```python
from build123d import *

# Parameters (mm, degrees)
BOSS_EXTRUDE1_DEPTH = 10
SKETCH4_R           = 1.75
CUT_EXTRUDE3_DEPTH  = 10
SKETCH6_R           = 2
CUT_EXTRUDE5_DEPTH  = 2
CUT_EXTRUDE6_DEPTH  = 29.447319733
SKETCH8_W           = 5
SKETCH8_H           = 4.5
SKETCH8_W_2         = 1
SKETCH8_H_2         = 7
CUT_EXTRUDE7_DEPTH  = 5
CUT_EXTRUDE8_DEPTH  = 9
FILLET6_R           = 0.5


with BuildPart() as part:
    # Sketch1 → Boss-Extrude1 (new body)
    with BuildSketch(Plane(origin=(0, 0, 0), x_dir=(1, 0, 0), z_dir=(0, 1, 0))):
        Polygon((0, 0), (17, 0), (17, -20.5), (12, -20.5), (12, -16), (1, -16), (1, -7), (0, -7), align=None)
    extrude(amount=BOSS_EXTRUDE1_DEPTH)

    # Sketch4 → Cut-Extrude3 (cut)
    with BuildSketch(Plane(origin=(0, 10, 0), x_dir=(1, 0, 0), z_dir=(0, 1, 0))):
        with Locations(Location((6, -11, 0), (0, 0, 270))):
            Circle(SKETCH4_R)
    extrude(amount=-CUT_EXTRUDE3_DEPTH, mode=Mode.SUBTRACT)

    # Sketch6 → Cut-Extrude5 (cut)
    with BuildSketch(Plane(origin=(0, 10, 0), x_dir=(1, 0, 0), z_dir=(0, 1, 0))):
        with Locations(Location((6, -11, 0), (0, 0, 270))):
            Circle(SKETCH6_R)
    extrude(amount=-CUT_EXTRUDE5_DEPTH, mode=Mode.SUBTRACT)

    # Sketch7 → Cut-Extrude6 (cut, through all)
    with BuildSketch(Plane.XZ):
        with BuildLine():
            Line((0, 10), (1, 10))
            ThreePointArc((1, 10), (2.5, 8.5), (1, 7))
            Line((1, 7), (0, 7))
            ThreePointArc((0, 7), (-1.5, 8.5), (0, 10))
        make_face()
        with BuildLine():
            Line((9, 16), (9, 20.5))
            ThreePointArc((9, 20.5), (10.5, 22), (12, 20.5))
            Line((12, 20.5), (12, 16))
            ThreePointArc((12, 16), (10.5, 14.5), (9, 16))
        make_face()
    extrude(amount=-CUT_EXTRUDE6_DEPTH, mode=Mode.SUBTRACT)

    # Sketch8 → Cut-Extrude7 (cut)
    with BuildSketch(Plane(origin=(0, 10, 0), x_dir=(1, 0, 0), z_dir=(0, 1, 0))):
        with Locations((14.5, -18.25)):
            Rectangle(SKETCH8_W, SKETCH8_H)
        with Locations((0.5, -3.5)):
            Rectangle(SKETCH8_W_2, SKETCH8_H_2)
    extrude(amount=-CUT_EXTRUDE7_DEPTH, mode=Mode.SUBTRACT)

    # Sketch9 → Cut-Extrude8 (cut)
    with BuildSketch(Plane(origin=(0, 10, 0), x_dir=(1, 0, 0), z_dir=(0, 1, 0))):
        with BuildLine():
            Line((8.35, -5.15), (0, -5.15))
            ThreePointArc((0, -5.15), (-1.65, -3.5), (0, -1.85))
            Line((0, -1.85), (8.35, -1.85))
            ThreePointArc((8.35, -1.85), (10, -3.5), (8.35, -5.15))
        make_face()
    extrude(amount=-CUT_EXTRUDE8_DEPTH, mode=Mode.SUBTRACT)

    # Fillet6
    fillet6_edges = [part.edges().sort_by_distance(p)[0] for p in [
        (0, 3, 1.85),
        (0, 3, 5.15),
        (1, 5, 16),
        (17, 5, 0),
        (17, 2.5, 20.5),
        (12, 2.5, 20.5),
        (0, 2.5, 7),
        (0, 2.5, 0),
    ]]
    fillet(fillet6_edges, radius=FILLET6_R)


solid = part.part
```
Source: CAD feature listing. Evaluate the final solid. Frame: model axes, mm. A direction names the side the tool comes from. Round coordinates to 2 decimals unless told otherwise and drop trailing zeros. Write each loop counter-clockwise with the first axis right and the second up, starting at its lowest first coordinate (ties: lowest second). Pieces come first, ordered by that corner, then holes. Notation, with made-up numbers: M -27,50 L 28,50 A28 ccw 28,74 Z; hole C 78.25,-5 d1. An arc over 180 degrees is marked long. Answer as a JSON object with one key per item and string values. Group by question number.
(1) Section query D-D on x = 16.25. Output: boundary loops of the cut face in (y, z), then the cut area to 4 significant figures.
(2) Section query B-B on z = 11.5. Output: boundary loops of the cut face in (x, y), then the cut area to 3 significant figures.
(3) Section query A-A on x = 6. Output: boundary loops of the cut face in (y, z).
(4) Ray query, line 1 (X direction, y = 9.65, z = 11); line 2 (Z direction, x = 5.75, y = 9); line 3 (X direction, y = 6.5, z = 11). Return the intervals inside material, ascending. Write a range as [from, to].
(5) Reachability of faces 5 (the flat face through (0.5, 5, 0.9)), 6 (the flat face through (14, 8, 16)), 7 (the cylindrical face through (6, 9, 9)) from +Z, -Z, +X, -X, +Y, -Y: full face, straight path, thin tool, end or side. Return the list, or none.
(6) Section query C-C on y = 6. Output: boundary loops of the cut face in (x, z), then the cut area to 3 significant figures.
(7) Mould query, pull axis Z, two halves, no side actions, for faces 1 (the flat face through (15, 2, 20.5)), 2 (the flat face through (4, 6, 1.85)), 3 (the flat face through (14, 5, 18)), 4 (the cylindrical face through (10, 5.6, 3.5)). Classes: +Z half, -Z half, draft (parallel to the pull), parting line (faces both ways), or undercut.
(8) First-contact query: pin 1 (3.5 mm diameter, centred on x = 4.5, z = 4, fed in from +Y); pin 2 (0.6 mm diameter, centred on y = 7, z = 6, fed in from -X); pin 3 (0.8 mm diameter, centred on x = 0.5, z = 1, fed in from +Y); pin 4 (6 mm diameter, centred on x = 6.5, y = 2.5, fed in from +Z). Flat tips, straight axial feed; report the tip coordinate or a pass-through.
Computed values:
{
 "1": {"outline": "M 0,0 L 10,0 L 10,16 L 5,16 L 5,20.5 L 0,20.5 Z", "area": "182.5 mm^2"},
 "2": {"outline": "M 1,0 L 4.32,0 L 4.32,8 L 4.06,8 L 4.06,10 L 1,10 Z; M 7.68,0 L 17,0 L 17,10 L 7.94,10 L 7.94,8 L 7.68,8 Z", "area": "125 mm^2"},
 "3": {"outline": "M 0,0 L 10,0 L 10,1.85 L 1,1.85 L 1,5.15 L 10,5.15 L 10,9 L 8,9 L 8,9.25 L 0,9.25 Z; M 0,12.75 L 8,12.75 L 8,13 L 10,13 L 10,16 L 0,16 Z"},
 "4": {"line 1": "[1, 4], [8, 17]", "line 2": "[0, 1.85], [5.15, 9.02], [12.98, 16]", "line 3": "[1, 4.25], [7.75, 17]"},
 "5": {"face 5": "+Z, -Z, -X, +Y", "face 6": "+Z, +X, -X, +Y", "face 7": "+Y"},
 "6": {"outline": "M 1,0 L 16.5,0 A0.5 ccw 17,0.5 L 17,16 L 12,16 A1.5 cw 9,16 L 1.5,16 A0.5 ccw 1,15.5 L 1,10 A1.5 cw 1,7 L 1,5.15 L 8.35,5.15 A1.65 cw 8.35,1.85 L 1,1.85 Z; hole C 6,11 d3.5", "area": "211 mm^2"},
 "7": {"face 1": "+Z half", "face 2": "undercut", "face 3": "draft", "face 4": "undercut"},
 "8": {"pin 1": "y = 10", "pin 2": "x = 1", "pin 3": "y = 5", "pin 4": "z = 16"}
}
